For this review, take the finished solid that the model builds, in its own axes (mm). A direction names the side the tool comes from. Coordinates: 2 decimals unless noted, no trailing zeros. Write each loop counter-clockwise with the first axis right and the second up, starting at its lowest first coordinate (ties: lowest second). Pieces come first, ordered by that corner, then holes. Notation, with made-up numbers: (51, -18.75) -> (73, -18.75) arc R20 ccw to (73, -9.75) -> close; hole circle Ø7 at (86.25, -36). An arc over 180 degrees is marked (long way). One line per item, written item: value. Start each with the question number.
1) Machinability: for faces 1 (the flat face through (-9, -15, 0)), 2 (the cylindrical face through (9.139, -14.334, 7.888)), which of the approach directions +Z, -Z, +X, -X, +Y, -Y give a long, thin tool a straight path to every point of the face, cutting with its end or side? Answer none if there is none.
2) Add section D-D (z = 13). State the section outline as (x, y) points.
3) For probe 1 along Y at (x, z) = (0, 9); probe 2 along X at (y, z) = (-5, 10.75); probe 3 along X at (y, z) = (-5.5, 3.75), list the stretches that pass through material, from the lowest coordinate up. Write a range as from..to.
4) For pin 1 Ø10 at (x, z) = (-6.5, 12) entering from +Y; pin 2 Ø4 at (x, z) = (-16, 9.5) entering from +Y; pin 3 Ø2 at (y, z) = (15.5, 16.5) entering from +X (3 decimals), all flat-tipped, find the tip position at first contact; note any pin that passes through.
5) Mouldability with a two-part tool opening along Y and no side actions: class faces 3 (the flat face through (0, 0, 19)), 4 (the cylindrical face through (-4.336, -19.524, 8.874)), 5 (the flat face through (0, 0, 16)) as released by +Y, released by -Y, zero draft, split by the parting line, or undercut.
6) Add section C-C (z = 17.25). State the section outline as (x, y) points, and give its area (3 significant figures).
7) Add section A-A (y = 0). State the section outline as (x, z) points, and give its area (3 significant figures).
from build123d import *

# Parameters (mm, degrees)
SKETCH_R        = 20
PAD_DEPTH       = 19
SKETCH001_R     = 17
POCKET_DEPTH    = 16
CHAMFER001_SIZE = 1


with BuildPart() as part:
    # Sketch → Pad (new body)
    with BuildSketch(Plane.XY):
        Circle(SKETCH_R)
    extrude(amount=PAD_DEPTH)

    # Sketch001 (on Face2 of Pad) → Pocket (cut)
    with BuildSketch(Plane(origin=(0, 0, 0), x_dir=(1, 0, 0), z_dir=(0, 0, -1))):
        Circle(SKETCH001_R)
    extrude(amount=-POCKET_DEPTH, mode=Mode.SUBTRACT)

    # Chamfer001
    chamfer001_edges = [part.edges().sort_by_distance(p)[0] for p in [
        (-20, 0, 19),
    ]]
    chamfer(chamfer001_edges, length=CHAMFER001_SIZE)


solid = part.part
Numbers:
1. face 1: -Z, +X, -X, +Y, -Y
1. face 2: -Z
2. outline: circle Ø40 at (0, 0); hole circle Ø34 at (0, 0)
3. probe 1: -20..-17, 17..20
3. probe 2: -19.36..-16.25, 16.25..19.36
3. probe 3: -19.23..-16.09, 16.09..19.23
4. pin 1: y = 19.94
4. pin 2: y = 14.28
4. pin 3: x = 13.775
5. face 3: zero draft
5. face 4: split by the parting line
5. face 5: undercut
6. outline: circle Ø40 at (0, 0)
6. area: 1,260 mm²
7. outline: (-20, 0) -> (-17, 0) -> (-17, 16) -> (17, 16) -> (17, 0) -> (20, 0) -> (20, 18) -> (19, 19) -> (-19, 19) -> (-20, 18) -> close
7. area: 215 mm²
